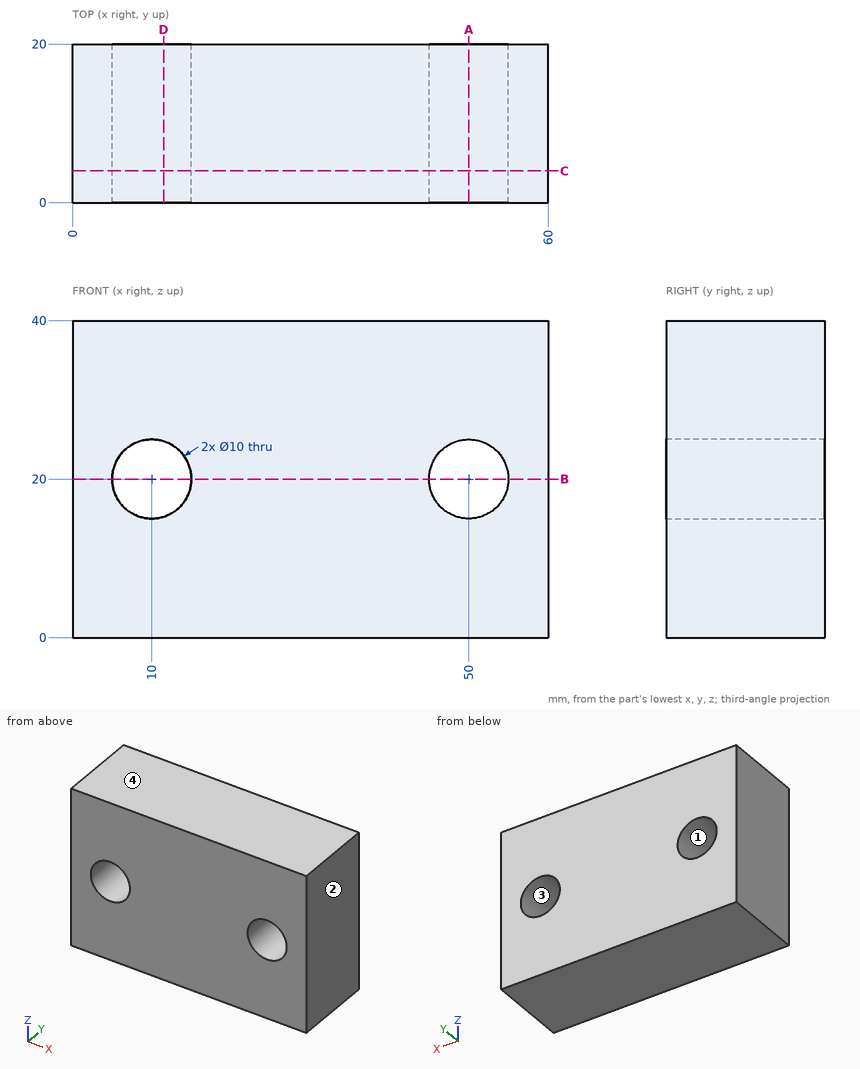
Job drawing, mm, ordinate dimensions from the low corner. One solid piece. Coordinates: 2 decimals unless noted, no trailing zeros. Order: outer loops, then holes, each group sorted by start corner. A loop starts at its lowest first (then second) coordinate and runs counter-clockwise, first axis right, second up. Notation, with made-up numbers: (45, -8) -> (58, -8) arc R15 ccw to (58, 0) -> close; hole circle Ø11 at (-18.75, 55). An arc over 180 degrees is marked (long way). Answer in a Markdown table with one row per item. Add a question column.
Q1. Wall check: line 1 along X through (y, z) = (4.5, 20); line 2 along Z through (x, y) = (10, 13.5); line 3 along X through (y, z) = (11.25, 21). Give the ranges that are in metal, low to high. Write a range as [from, to].
Q2. Drop a flat-ended pin along its axis: pin 1 (6 mm diameter, centred on x = 50, z = 20, fed in from -Y). Give the stop position or say it passes through.
Q3. Mould opens along Z. For the marked faces 1, 2, 3 and 4 say: +Z half, -Z half, draft (parallel to the pull), parting line (faces both ways), or undercut.
Q4. Band-saw the part on D-D, the plane x = 11.5. List the corners of the cut face in (y, z).
Q5. Band-saw the part on A-A, the plane x = 50. List the corners of the cut face in (y, z).
Q6. Band-saw the part on B-B, the plane z = 20. List the corners of the cut face in (x, y).
Q7. Band-saw the part on C-C, the plane y = 4. List the corners of the cut face in (x, z).
Answers follow:
| question | item | result |
|---|---|---|
| 1 | line 1 | [0, 5], [15, 45], [55, 60] |
| 1 | line 2 | [0, 15], [25, 40] |
| 1 | line 3 | [0, 5.1], [14.9, 45.1], [54.9, 60] |
| 2 | pin 1 | through |
| 3 | face 1 | undercut |
| 3 | face 2 | draft |
| 3 | face 3 | undercut |
| 3 | face 4 | +Z half |
| 4 | outline | (0, 0) -> (20, 0) -> (20, 15.23) -> (0, 15.23) -> close; (0, 24.77) -> (20, 24.77) -> (20, 40) -> (0, 40) -> close |
| 5 | outline | (0, 0) -> (20, 0) -> (20, 15) -> (0, 15) -> close; (0, 25) -> (20, 25) -> (20, 40) -> (0, 40) -> close |
| 6 | outline | (0, 0) -> (5, 0) -> (5, 20) -> (0, 20) -> close; (15, 0) -> (45, 0) -> (45, 20) -> (15, 20) -> close; (55, 0) -> (60, 0) -> (60, 20) -> (55, 20) -> close |
| 7 | outline | (0, 0) -> (60, 0) -> (60, 40) -> (0, 40) -> close; hole circle Ø10 at (10, 20); hole circle Ø10 at (50, 20) |
